Answer from the drawing. Dimensions are ordinates in mm from the lowest x, y and z of the part. A direction names the side the tool comes from. Give positions to 0.01 mm unless a question says otherwise; leave off trailing zeros. Loops run counter-clockwise (first coordinate to the right, second up) from the corner with the lowest first, then second, coordinate; pieces in that order, holes last.
Item 1: Section A-A, the plane x = 70 is taken. Give the vertices of the cut face in (y, z).
Item 2: Section B-B, the plane y = 17.5 is taken. Give the vertices of the cut face in (x, z), and give its area (3 significant figures).
Item 3: Each of these flat-tipped pins is pushed along its axis until it touches: pin 1 Ø1.5 at (x, y) = (122.5, 2.5) entering from -Z; pin 2 Ø2.5 at (y, z) = (2.5, 15.5) entering from +X; pin 3 Ø2.5 at (x, y) = (19, 3) entering from -Z. Where does it stop, or does it pass through?
Item 4: Section D-D, the plane x = 55.5 is taken. Give the vertices of the cut face in (y, z).
Item 5: Consider line 1 along Z through (x, y) = (11.5, 39); line 2 along X through (y, z) = (15.5, 81.5); line 3 along X through (y, z) = (8.5, 38.5). Determine where each line is inside the solid, lowest interval first.
Item 6: A tool of negligible diameter and unlimited length cuts with its end or side. For the marked faces 4, 5 and 6, from which of +Z, -Z, +X, -X, +Y, -Y can it reach the whole face along a straight path? Write none if from no direction.
Item 7: The mould has two halves that part along X. Classify the marked faces 1, 2 and 3: pulls with the +X half, pulls with the -X half, needs draft (parallel to the pull), parting line crosses it, or undercut.
Item 8: Section C-C, the plane z = 38.5 is taken. Give the vertices of the cut face in (x, y).
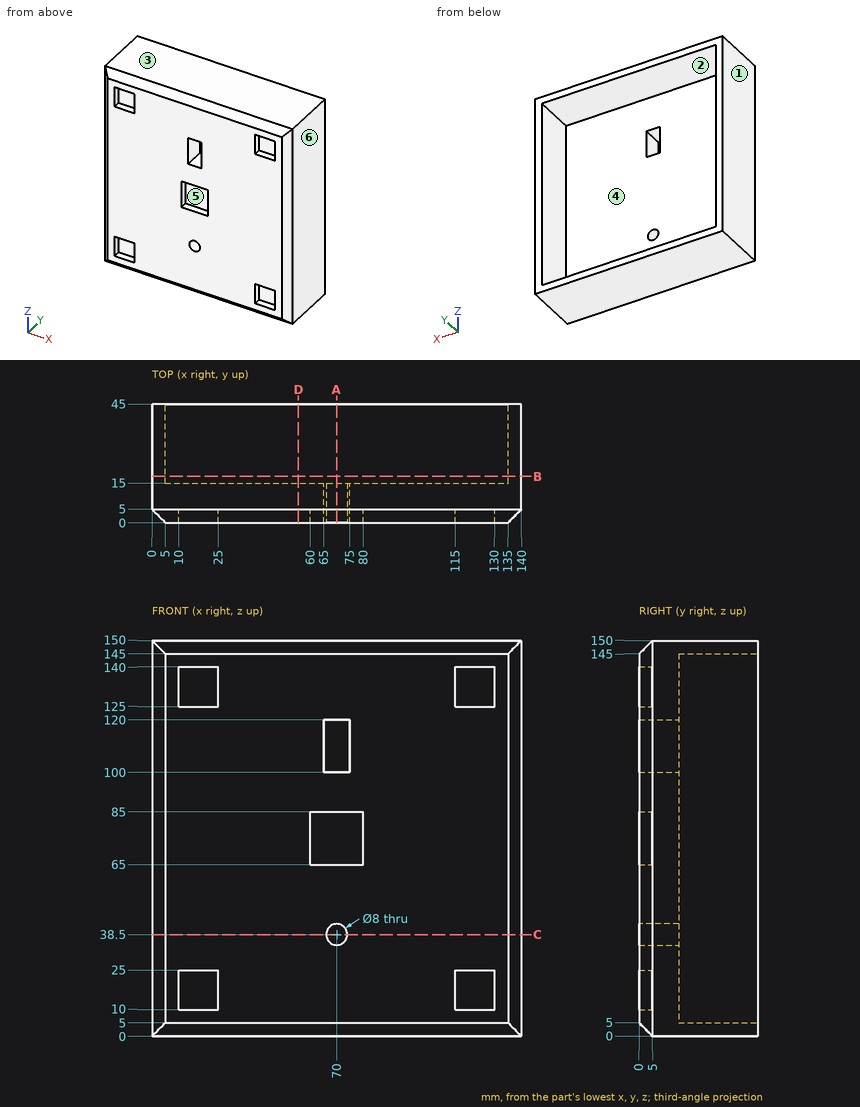
Worked answers:
1. outline: (0, 5) - (5, 0) - (45, 0) - (45, 5) - (15, 5) - (15, 34.5) - (0, 34.5) - close; (0, 42.5) - (15, 42.5) - (15, 100) - (0, 100) - (0, 85) - (5, 85) - (5, 65) - (0, 65) - close; (0, 120) - (15, 120) - (15, 145) - (45, 145) - (45, 150) - (5, 150) - (0, 145) - close
2. outline: (0, 0) - (140, 0) - (140, 150) - (0, 150) - close; hole (5, 5) - (135, 5) - (135, 145) - (5, 145) - close
2. area: 2,800 mm2
3. pin 1: stops at z = 1.75
3. pin 2: stops at x = 138.75
3. pin 3: stops at z = 0.75
4. outline: (0, 5) - (5, 0) - (45, 0) - (45, 5) - (15, 5) - (15, 145) - (45, 145) - (45, 150) - (5, 150) - (0, 145) - close
5. line 1: z = 0 to 5, 145 to 150
5. line 2: x = 0 to 5, 135 to 140
5. line 3: x = 0 to 66, 74 to 140
6. face 4: +Y
6. face 5: -Y
6. face 6: +Z, -Z, +X, +Y, -Y
7. face 1: pulls with the -X half
7. face 2: undercut
7. face 3: needs draft
8. outline: (0, 5) - (5, 0) - (66, 0) - (66, 15) - (5, 15) - (5, 45) - (0, 45) - close; (74, 0) - (135, 0) - (140, 5) - (140, 45) - (135, 45) - (135, 15) - (74, 15) - close
